Design review of the part built by this model. Coordinates are the model's own, in mm. A direction names the side the tool comes from. Give positions to 0.01 mm unless a question says otherwise; leave off trailing zeros. Order: outer loops, then holes, each group sorted by start corner. A loop starts at its lowest first (then second) coordinate and runs counter-clockwise, first axis right, second up.
```python
from build123d import *

# Parameters (mm, degrees)
ESQUISSE1_W             = 12
ESQUISSE1_H             = 108
ESQUISSE1_W_2           = 100
ESQUISSE1_H_2           = 12
BOSS_EXTRU_1_DEPTH      = 120
ESQUISSE2_RX            = 42.771597922
ESQUISSE2_RY            = 10
ENL_V_MAT_EXTRU_1_DEPTH = 12
CONG_1_R                = 10
CONG_2_R                = 10
CONG_3_R                = 2
CONG_4_R                = 2
CONG_5_R                = 2


with BuildPart() as part:
    # Esquisse1 → Boss.-Extru.1 (new body)
    with BuildSketch(Plane.XY):
        with Locations((6, 66)):
            Rectangle(ESQUISSE1_W, ESQUISSE1_H)
        with Locations((50, 6)):
            Rectangle(ESQUISSE1_W_2, ESQUISSE1_H_2)
    extrude(amount=-BOSS_EXTRU_1_DEPTH)

    # Esquisse2 → Enlèv. mat.-Extru.1 (cut)
    with BuildSketch(Plane.ZY):
        with Locations(Location((-60, 90), (0, 0, 0))):
            Ellipse(ESQUISSE2_RX, ESQUISSE2_RY)
    extrude(amount=-ENL_V_MAT_EXTRU_1_DEPTH, mode=Mode.SUBTRACT)

    # Congé1
    cong_1_edges = [part.edges().sort_by_distance(p)[0] for p in [
        (100, 12, -60),
    ]]
    fillet(cong_1_edges, radius=CONG_1_R)

    # Congé2
    cong_2_edges = [part.edges().sort_by_distance(p)[0] for p in [
        (12, 12, -60),
    ]]
    fillet(cong_2_edges, radius=CONG_2_R)

    # Congé3
    cong_3_edges = [part.edges().sort_by_distance(p)[0] for p in [
        (100, 1, 0),
        (97.071067812, 9.071067812, 0),
        (56, 12, 0),
        (12, 71, 0),
        (14.928932188, 14.928932188, 0),
    ]]
    fillet(cong_3_edges, radius=CONG_3_R)

    # Congé4
    cong_4_edges = [part.edges().sort_by_distance(p)[0] for p in [
        (100, 1, -120),
        (97.071067812, 9.071067812, -120),
        (56, 12, -120),
        (12, 71, -120),
        (14.928932188, 14.928932188, -120),
    ]]
    fillet(cong_4_edges, radius=CONG_4_R)

    # Congé5
    cong_5_edges = [part.edges().sort_by_distance(p)[0] for p in [
        (5, 120, 0),
        (5, 120, -120),
        (11.414213562, 120, -0.585786438),
        (12, 120, -60),
        (11.414213562, 120, -119.414213562),
    ]]
    fillet(cong_5_edges, radius=CONG_5_R)


solid = part.part
```
1. For pin 1 (3 mm diameter, centred on x = 84, z = -23, fed in from +Y), flat-tipped, find the tip position at first contact; note if it passes through.
Recorded:
pin 1: stops at y = 12
2. Take a section at C-C (z = -109). State the section outline as (x, y) points, then the cut area to 3 significant figures.
Recorded:
outline: (0, 0) - (100, 0) - (100, 2) arc R10 ccw to (90, 12) - (22, 12) arc R10 cw to (12, 22) - (12, 118) arc R2 ccw to (10, 120) - (0, 120) - close
area: 2,500 mm2
3. Machinability: for faces 1 (the face through (9, 37, 0)), 2 (the face through (12, 69, -59)), which of the approach directions +Z, -Z, +X, -X, +Y, -Y give a long, thin tool a straight path to every point of the face, cutting with its end or side? Answer none if there is none.
Recorded:
face 1: +Z, +X, -X, +Y, -Y
face 2: +Z, -Z, +X, +Y
4. Take a section at A-A (x = 84). State the section outline as (y, z) points.
Recorded:
outline: (0, -120) - (10, -120) arc R2 ccw to (12, -118) - (12, -2) arc R2 ccw to (10, 0) - (0, 0) - close
5. For line 1 along X through (y, z) = (52, -85.5); line 2 along Z through (x, y) = (8, 87), list the stretches that pass through material, from the lowest coordinate up.
Recorded:
line 1: x = 0 to 12
line 2: z = -120 to -100.8, -19.2 to 0
